Check sheet for the modelled part. Datum: model origin and axes. Units: mm. A direction names the side the tool comes from. Give positions to 0.01 mm unless a question says otherwise; leave off trailing zeros. Order: outer loops, then holes, each group sorted by start corner. A loop starts at its lowest first (then second) coordinate and runs counter-clockwise, first axis right, second up.
Item 1: Sectioned sample at A-A on x = 0. Record the boundary of the cut face in (y, z) (3 decimals).
Item 2: Material ranges on line 1 along Y through (x, z) = (0.1, 1.5); line 2 along X through (y, z) = (-1, -2.75); line 3 along X through (y, z) = (-1.7, 1), recorded low to high.
Item 3: Sectioned sample at D-D on z = 1. Record the boundary of the cut face in (x, y), and give its area (3 significant figures).
Item 4: Sectioned sample at C-C on z = -1.5. Record the boundary of the cut face in (x, y) (3 decimals).
Item 5: Access from +Z, -Z, +X, -X, +Y, -Y to the whole of each face (thin tool, end or side, straight path). Record for faces 1 (the flat face through (0, 0, 3.5)), 2 (the cylindrical face through (-1.873, -0.082, -1.662)).
from build123d import *

# Parameters (mm, degrees)
SKETCH017_R     = 2.25
PAD003_DEPTH    = 3.5
CHAMFER001_SIZE = 1
SKETCH020_R     = 1.875
PAD006_DEPTH    = 3.5
CHAMFER002_SIZE = 0.36
CHAMFER003_SIZE = 0.5


with BuildPart() as part:
    # Sketch017 → Pad003 (new body)
    with BuildSketch(Plane.XY):
        Circle(SKETCH017_R)
    extrude(amount=PAD003_DEPTH)

    # Chamfer001
    chamfer001_edges = [part.edges().sort_by_distance(p)[0] for p in [
        (-2.25, 0, 3.5),
    ]]
    chamfer(chamfer001_edges, length=CHAMFER001_SIZE)

    # Sketch020 (on Face3 of Chamfer001) → Pad006 (join)
    with BuildSketch(Plane(origin=(0, 0, 0), x_dir=(1, 0, 0), z_dir=(0, 0, -1))):
        Circle(SKETCH020_R)
    extrude(amount=PAD006_DEPTH)

    # Chamfer002
    chamfer002_edges = [part.edges().sort_by_distance(p)[0] for p in [
        (-1.875, 0, 0),
    ]]
    chamfer(chamfer002_edges, length=CHAMFER002_SIZE)

    # Chamfer003
    chamfer003_edges = [part.edges().sort_by_distance(p)[0] for p in [
        (-1.875, 0, -3.5),
    ]]
    chamfer(chamfer003_edges, length=CHAMFER003_SIZE)


solid = part.part
Report:
1. outline: (-2.25, 0) - (-2.235, 0) - (-1.875, -0.36) - (-1.875, -3) - (-1.375, -3.5) - (1.375, -3.5) - (1.875, -3) - (1.875, -0.36) - (2.235, 0) - (2.25, 0) - (2.25, 2.5) - (1.25, 3.5) - (-1.25, 3.5) - (-2.25, 2.5) - close
2. line 1: y = -2.25 to 2.25
2. line 2: x = -1.59 to 1.59
2. line 3: x = -1.47 to 1.47
3. outline: circle Ø4.5 at (0, 0)
3. area: 15.9 mm2
4. outline: circle Ø3.75 at (0, 0)
5. face 1: +Z, +X, -X, +Y, -Y
5. face 2: -Z
